```python
from build123d import *

# Parameters (mm, degrees)
M3_GEWINDEBOHRUNG1_D     = 2.5
M3_GEWINDEBOHRUNG1_DEPTH = 6.5
M3_GEWINDEBOHRUNG1_TIP   = 0.751075774
FASE1_SIZE               = 0.2


with BuildPart() as part:
    # Skizze1 → Rotation1 (revolve)
    with BuildSketch(Plane.XY, mode=Mode.PRIVATE) as rotation1_sk:
        Polygon((19, 0), (-16, 0), (-16, 2), (16, 2), (16, 1.25), (19, 1.25), align=None)
    revolve(rotation1_sk.sketch.rotate(Axis((0, 0, 0), (1, 0, 0)), 90), axis=Axis((0, 0, 0), (1, 0, 0)))

    # M3 Gewindebohrung1
    with Locations(Plane.ZY.offset(16)):
        with Locations((0, 0)):
            Hole(M3_GEWINDEBOHRUNG1_D / 2, depth=M3_GEWINDEBOHRUNG1_DEPTH)
            with Locations((0, 0, -(M3_GEWINDEBOHRUNG1_DEPTH + M3_GEWINDEBOHRUNG1_TIP / 2))):  # 118° drill point
                Cone(0, M3_GEWINDEBOHRUNG1_D / 2, M3_GEWINDEBOHRUNG1_TIP, mode=Mode.SUBTRACT)

    # Fase1
    fase1_edges = [part.edges().sort_by_distance(p)[0] for p in [
        (19, 0, -1.25),
    ]]
    chamfer(fase1_edges, length=FASE1_SIZE)


solid = part.part
```
Geometry: final body of the model. Coordinates: model frame, mm. A direction names the side the tool comes from. Round coordinates to 2 decimals unless told otherwise and drop trailing zeros. Loops run counter-clockwise (first coordinate to the right, second up) from the corner with the lowest first, then second, coordinate; pieces in that order, holes last.
Item 1: Mould query, pull axis Y, two halves, no side actions, for faces 1 (the flat face through (-16, -1, -1)), 2 (the cylindrical face through (17.42, -0.05, -1.25)), 3 (the cylindrical face through (-12.7, -1.22, 0.27)). Classes: released by +Y, released by -Y, zero draft, split by the parting line, or undercut.
Checked values:
face 1: zero draft
face 2: split by the parting line
face 3: undercut
Item 2: Section B-B, the plane y = 1.7. Output: boundary loops of the cut face in (x, z).
Checked values:
outline: (-16, -1.05) - (16, -1.05) - (16, 1.05) - (-16, 1.05) - close
Item 3: Reachability of faces 4 (the flat face through (16, -1, 1)), 5 (the flat face through (19, 0, 0)) from +Z, -Z, +X, -X, +Y, -Y: full face, straight path, thin tool, end or side. Return the list, or none.
Checked values:
face 4: +X
face 5: +Z, -Z, +X, +Y, -Y
Item 4: Line query: L1, parallel to Y at x = -10.75, z = 0; L2, parallel to X at y = -1.3, z = -0.55; L3, parallel to Z at x = -14, y = 0.5. Output: solid intervals per line, ascending.
Checked values:
L1: y = -2 to -1.25, 1.25 to 2
L2: x = -16 to 16
L3: z = -1.94 to -1.15, 1.15 to 1.94
Item 5: Contact query for flat-ended pins moving along their axis: P1, Ø2, axis at y = 0, z = 0, coming from the -X side; P2, Ø1, axis at x = -7, z = -0.5, coming from the -Y side; P3, Ø1.5, axis at x = 6.5, y = -1.5, coming from the +Z side. Output: stop coordinate, or through.
Checked values:
P1: stops at x = -9.35
P2: stops at y = -2
P3: stops at z = 1.85
Item 6: Section A-A, the plane x = -0.5. Output: boundary loops of the cut face in (y, z), plus the area to 3 significant figures.
Checked values:
outline: circle Ø4 at (0, 0)
area: 12.6 mm2
